Geometry: final body of the model. Coordinates: model frame, mm. Give positions to 0.01 mm unless a question says otherwise; leave off trailing zeros.
Q1. Line query: L1, parallel to Y at x = -22.5, z = 3.1; L2, parallel to X at y = 47, z = 4.15; L3, parallel to X at y = 48.5, z = 3.25. Output: solid intervals per line, ascending.
Q2. Pin query (flat end, axial travel): pin 1 (1.5 mm diameter, centred on x = -33.5, z = 4.5, fed in from -Y); pin 2 (3 mm diameter, centred on y = 35.5, z = 4.5, fed in from +X); pin 3 (1.5 mm diameter, centred on x = -41, y = 41, fed in from +Z). Return the tip coordinate at first contact, or that it passes through.
Q3. Draft query along Y for faces 1 (the face through (-26.191, 53.696, 2.868)), 2 (the face through (-26, 36, 0)), 3 (the face through (-27.102, 43.256, 2.504)). Return one class per face: pulls with the +Y half, pulls with the -Y half, needs draft (parallel to the pull), parting line crosses it, or undercut.
```python
from build123d import *

# Parameters (mm, degrees)
F0_W        = 37.4135075825
F0_H        = 37.4135057104
F0_R        = 5.08
F1_DEPTH    = 5.08
F2_R        = 5.07999
F3_R        = 5.07999
F4_T1_DEPTH = 57.7335175825
F4_T3_DEPTH = 25.40001
F4_T6_ANGLE = 90
F5_R        = 5.07999


# Not quite as in the source:
# - a fillet or chamfer that OpenCascade refuses, or shapes differently, is made with other operations: its cross-section is extruded or revolved along the edge and cut away or added
# - a fillet or chamfer is up to 0.001 mm smaller than in the source, because OpenCascade refuses the exact size


with BuildPart() as f1:
    # F0 (on Top) → F1 (new body)
    with BuildSketch(Plane.XY):
        with Locations((-26.0004317388, 35.8758829534)):
            Rectangle(F0_W, F0_H)
        with Locations((-26.0004317388, 48.2149645656)):
            Circle(F0_R, mode=Mode.SUBTRACT)
    extrude(amount=F1_DEPTH)

    # F2 (radius 5.08 in the source; OpenCascade refuses exactly that, so slightly less here)
    f2_edges = [f1.edges().sort_by_distance(p)[0] for p in [
        (-26.000432, 17.16913, 5.08),
    ]]
    fillet(f2_edges, radius=F2_R)

    # F3 (radius 5.08 in the source; OpenCascade refuses exactly that, so slightly less here)
    f3_edges = [f1.edges().sort_by_distance(p)[0] for p in [
        (-7.293678, 38.415878, 5.08),
    ]]
    fillet(f3_edges, radius=F3_R)

    # F4: fillet of radius 5.08 on 1 edges, made by hand

    # F4_s2 → F4_t1 (cut)
    with BuildSketch(Plane.YZ.offset(-57.40718553)):
        with BuildLine():
            ThreePointArc((54.5826358086, 0), (53.094738257, 3.5921024484), (49.5026358086, 5.08))
            Line((49.5026358086, 5.08), (54.5826358086, 5.08))
            Line((54.5826358086, 5.08), (54.5826358086, 0))
        make_face()
    extrude(amount=F4_T1_DEPTH, mode=Mode.SUBTRACT)

    # F4_s4 → F4_t3 (cut)
    with BuildSketch(Plane.XY.offset(-12.7)):
        with BuildLine():
            ThreePointArc((-7.2936779475, 49.5026358086), (-8.7815754991, 53.094738257), (-12.3736779475, 54.5826358086))
            Line((-12.3736779475, 54.5826358086), (-7.2936779475, 54.5826358086))
            Line((-7.2936779475, 54.5826358086), (-7.2936779475, 49.5026358086))
        make_face()
    extrude(amount=F4_T3_DEPTH, mode=Mode.SUBTRACT)

    # F4_s5 → F4_t6 (revolve, cut)
    with BuildSketch(Plane.XY.offset(1e-05)):
        with BuildLine():
            ThreePointArc((-12.3736679475, 54.5826358086), (-8.7815719636, 53.0947347215), (-7.2936779475, 49.5026358086))
            Line((-7.2936779475, 49.5026358086), (-7.2936779475, 54.5826358086))
            Line((-7.2936779475, 54.5826358086), (-12.3736679475, 54.5826358086))
        make_face()
    revolve(axis=Axis((-12.3736679475, 54.5826358086, 1e-05), (0, -1, 0)), revolution_arc=F4_T6_ANGLE, mode=Mode.SUBTRACT)

    # F5 (radius 5.08 in the source; OpenCascade refuses exactly that, so slightly less here)
    f5_edges = [f1.edges().sort_by_distance(p)[0] for p in [
        (-44.707186, 35.875878, 5.08),
        (-44.707186, 17.16913, 5e-06),
        (-44.707186, 18.657025, 3.592105),
        (-44.707186, 53.094738, 3.592102),
    ]]
    fillet(f5_edges, radius=F5_R)


solid = f1.part
```
Data:
1. L1: y = 18.22 to 44.53, 51.9 to 53.53
1. L2: x = -42.56 to -30.93, -21.07 to -9.44
1. L3: x = -43.53 to -31.07, -20.93 to -8.47
2. pin 1: stops at y = 18.82
2. pin 2: stops at x = -8.27
2. pin 3: stops at z = 5.04
3. face 1: pulls with the +Y half
3. face 2: needs draft
3. face 3: undercut
